The model under review builds one solid part; all positions refer to its coordinate system, in mm. A direction names the side the tool comes from. Coordinates: 2 decimals unless noted, no trailing zeros. Write each loop counter-clockwise with the first axis right and the second up, starting at its lowest first coordinate (ties: lowest second). Pieces come first, ordered by that corner, then holes. Notation, with made-up numbers: M -34.5,-23.5 L -21.5,-23.5 A8 cw -21.5,-10.5 Z; hole C 22.25,43.25 d1. An arc over 180 degrees is marked long. Answer as CSV lines item,"result". Start each with the question number.
from build123d import *

# Parameters (mm, degrees)
SKETCH_1_R      = 1.65
EXTRUDE_1_DEPTH = 47
SKETCH_3_R      = 11
EXTRUDE_2_DEPTH = 2
EXTRUDE_3_DEPTH = 22


with BuildPart() as part:
    # 草图1 → 凸台-拉伸1 (new body)
    with BuildSketch(Plane.XY):
        Polygon((-21.15, 16.15), (-16.15, 21.15), (16.15, 21.15), (21.15, 16.15), (21.15, -16.15), (16.15, -21.15), (-16.15, -21.15), (-21.15, -16.15), align=None)
        with Locations((15.5, 15.5)):
            Circle(SKETCH_1_R, mode=Mode.SUBTRACT)
        with Locations((-15.5, 15.5)):
            Circle(SKETCH_1_R, mode=Mode.SUBTRACT)
        with Locations((15.5, -15.5)):
            Circle(SKETCH_1_R, mode=Mode.SUBTRACT)
        with Locations((-15.5, -15.5)):
            Circle(SKETCH_1_R, mode=Mode.SUBTRACT)
    extrude(amount=EXTRUDE_1_DEPTH)

    # 草图3 → 凸台-拉伸2 (add)
    with BuildSketch(Plane(origin=(0, 0, 0), x_dir=(-1, 0, 0), z_dir=(0, 0, -1))):
        Circle(SKETCH_3_R)
    extrude(amount=EXTRUDE_2_DEPTH)

    # 草图4 → 凸台-拉伸3 (add)
    with BuildSketch(Plane(origin=(0, 0, -2), x_dir=(-1, 0, 0), z_dir=(0, 0, -1))):
        with BuildLine():
            Line((-1.5, 2), (1.5, 2))
            ThreePointArc((1.5, 2), (0, -2.5), (-1.5, 2))
        make_face()
    extrude(amount=EXTRUDE_3_DEPTH)


solid = part.part
1) Take a section at B-B on y = 0. Give the boundary of the cut face in (x, z), and give its area (3 significant figures).
2) Mouldability with a two-part tool opening along X and no side actions: class faces 4 (the flat face through (18.7, -18.6, 23.2)), 5 (the cylindrical face through (-13.976, 14.868, 23.171)), 6 (the flat face through (-18.6, -18.7, 23.2)) as +X half, -X half, draft (parallel to the pull), parting line (faces both ways), or undercut.
3) Take a section at D-D on z = -18. Give the boundary of the cut face in (x, y), and give its area (3 significant figures).
4) Clearance check with flat-ended pins moving along their axes: pin 1 Ø3 at (x, y) = (-16.5, 0) entering from -Z; pin 2 Ø2.5 at (x, z) = (0.5, -14) entering from +Y. State where each tip first meets the part, or that it passes through.
5) Take a section at C-C on x = 15. Give the boundary of the cut face in (y, z).
6) Take a section at A-A on x = 0. Give the boundary of the cut face in (y, z).
7) To check wall thickness, follow line 1 (Y direction, x = 15.5, z = 22); line 2 (X direction, y = 15, z = 25); line 3 (Y direction, x = 17, z = 7). State the ranges of each line that lie inside material, in increasing order. Write a range as [from, to].
8) Tool access review of faces 1 (the flat face through (0, 2, -13)), 2 (the flat face through (-9, -9, 0)), 3 (the cylindrical face through (17.024, 14.868, 23.171)): name each direction out of +Z, -Z, +X, -X, +Y, -Y from which nothing blocks a thin tool from reaching the whole face with its end or side.
Results:
1,outline,"M -21.15,0 L -11,0 L -11,-2 L -2.5,-2 L -2.5,-24 L 2.5,-24 L 2.5,-2 L 11,-2 L 11,0 L 21.15,0 L 21.15,47 L -21.15,47 Z"
1,area,"2,140 mm²"
2,face 4,"+X half"
2,face 5,"undercut"
2,face 6,"-X half"
3,outline,"M -1.5,2 A2.5 ccw long 1.5,2 Z"
3,area,"18.6 mm²"
4,pin 1,"stops at z = 0"
4,pin 2,"stops at y = 2"
5,outline,"M -21.15,0 L -17.07,0 L -17.07,47 L -21.15,47 Z; M -13.93,0 L 13.93,0 L 13.93,47 L -13.93,47 Z; M 17.07,0 L 21.15,0 L 21.15,47 L 17.07,47 Z"
6,outline,"M -21.15,0 L -11,0 L -11,-2 L -2.5,-2 L -2.5,-24 L 2,-24 L 2,-2 L 11,-2 L 11,0 L 21.15,0 L 21.15,47 L -21.15,47 Z"
7,line 1,"y = [-21.15, -17.15], [-13.85, 13.85], [17.15, 21.15]"
7,line 2,"x = [-21.15, -17.07], [-13.93, 13.93], [17.07, 21.15]"
7,line 3,"y = [-20.3, -16.19], [-14.81, 14.81], [16.19, 20.3]"
8,face 1,"-Z, +X, -X, +Y"
8,face 2,"-Z"
8,face 3,"+Z, -Z"
